Design review of the part built by this model. Coordinates are the model's own, in mm. A direction names the side the tool comes from. Round coordinates to 2 decimals unless told otherwise and drop trailing zeros. Order: outer loops, then holes, each group sorted by start corner. A loop starts at its lowest first (then second) coordinate and runs counter-clockwise, first axis right, second up.
Autodesk Inventor part; units mm, degrees
ref_plane "YZ Plane" through (0, 0, 0) normal (1, 0, 0) x (0, 1, 0)
ref_plane "XZ Plane" through (0, 0, 0) normal (0, 1, 0) x (-1, 0, 0)
ref_plane "XY Plane" through (0, 0, 0) normal (0, 0, 1) x (1, 0, 0)
sketch "Sketch1" plane through (0, 0, 0) normal (0, 0, 1) x (1, 0, 0)
  circle A0 centre (0, 0) radius 3.615
  circle A1 centre (0, 0) radius 5
  dimension "d0" = 7.23
  dimension "d1" = 10
sketch "Sketch2" plane through (0, 0, 0) normal (0, 0, 1) x (1, 0, 0)
  line L0 (5.0177, 0) -> (5.0177, 4.7273)
  line L1 (5.0177, 0) -> (9.745, 0) construction
  line L2 (5.0177, 4.7273) -> (5.0177, -3.9213)
  point P0 (0, 0)
  dimension "d2" = 90
revolve "Revolution1" add sketch "Sketch1" angle 90 about axis through (5.0177, 0, 0) along (0, 1, 0)
sketch "Sketch3" plane through (5.0177, 0, 5.0177) normal (1, 0, 0) x (0, 0, -1)
  point P0 (5.0177, 0)
sketch "Sketch4" plane through (5.0177, 0, 5.0177) normal (1, 0, 0) x (0, 0, -1)
  circle A0 centre (0, 0) radius 3.615
  circle A1 centre (0, 0) radius 5
  point P0 (5.0177, 0)
  dimension "d4" = 7.23
  dimension "d5" = 10
extrude "Extrusion1" add sketch "Sketch4" along normal blind 15
sketch "Sketch5" plane through (0, 0, 0) normal (0, 0, -1) x (-1, 0, 0)
  circle A0 centre (0, 0) radius 3.615
  circle A1 centre (0, 0) radius 5
  dimension "d8" = 7.23
  dimension "d9" = 10
extrude "Extrusion2" add sketch "Sketch5" along normal blind 15
properties part number "Knee-big"
1) Clearance check with flat-ended pins moving along their axes: P1, Ø6, axis at x = 0, y = 0, coming from the +Z side; P2, Ø5, axis at y = 3.5, z = 0.5, coming from the -X side; P3, Ø4, axis at x = -1, z = -11, coming from the +Y side; P4, Ø1.5, axis at y = -2.5, z = -10.5, coming from the +X side. State where each tip first meets the part, or that it passes through.
Results:
P1: stops at z = 9.81
P2: stops at x = -4.89
P3: stops at y = 5
P4: stops at x = 4.68
2) For faces 4 (the face through (12.41, -0.16, 8.63)), 5 (the face through (1.08, 4.88, -7.4)), 6 (the face through (20.018, 3, 2)), list the 3-axis set-ups (+Z, -Z, +X, -X, +Y, -Y) from which the entire face can be reached by the end or side of a thin tool; tool diameter is ignored.
Results:
face 4: +X
face 5: -Z
face 6: +Z, -Z, +X, +Y, -Y
3) Take a section at C-C on x = 9.25. Give the boundary of the cut face in (y, z) (3 decimals), plus the area to 3 significant figures.
Results:
outline: circle Ø10 at (0, 5.018); hole circle Ø7.23 at (0, 5.018)
area: 37.5 mm2
4) Take a section at B-B on z = -4.5. Give the boundary of the cut face in (x, y) (3 decimals).
Results:
outline: circle Ø10 at (0, 0); hole circle Ø7.23 at (0, 0)
5) The part is to be moulded in two halves that separate along Y. For faces 1 (the face through (12.413, 3.042, 8.986)), 2 (the face through (-3.34, 1.38, -7.4)), 3 (the face through (-3, 3, -15)), say which applies: released by +Y, released by -Y, zero draft, split by the parting line, or undercut.
Results:
face 1: split by the parting line
face 2: undercut
face 3: zero draft
6) Take a section at D-D on y = -2.25. Give the boundary of the cut face in (x, z).
Results:
outline: (-4.47, -15) - (-2.83, -15) - (-2.83, 0) arc R7.85 cw to (5.02, 7.85) - (20.02, 7.85) - (20.02, 9.48) - (5.02, 9.48) arc R9.48 ccw to (-4.47, 0) - close; (2.83, -15) - (4.47, -15) - (4.47, 0) arc R0.55 cw to (5.02, 0.55) - (20.02, 0.55) - (20.02, 2.19) - (5.02, 2.19) arc R2.19 ccw to (2.83, 0) - close
7) To check wall thickness, follow line 1 along Y through (x, z) = (0, -11.5) (3 decimals); line 2 along X through (y, z) = (-2.25, -7.25). State the ranges of each line that lie inside material, in increasing order.
Results:
line 1: y = -5 to -3.615, 3.615 to 5
line 2: x = -4.47 to -2.83, 2.83 to 4.47
8) Take a section at A-A on y = 0. Give the boundary of the cut face in (x, z) (3 decimals).
Results:
outline: (-5, -15) - (-3.615, -15) - (-3.615, 0) arc R8.633 cw to (5.018, 8.633) - (20.018, 8.633) - (20.018, 10.018) - (5.018, 10.018) arc R10.018 ccw to (-5, 0) - close; (3.615, -15) - (5, -15) - (5, 0) arc R0.018 cw to (5.018, 0.018) - (20.018, 0.018) - (20.018, 1.403) - (5.018, 1.403) arc R1.403 ccw to (3.615, 0) - close
